CAD build for the part. Positions are in the model's coordinates, mm. A direction names the side the tool comes from. Give positions to 0.01 mm unless a question says otherwise; leave off trailing zeros. Answer as a JSON object with one key per item and string values.
from build123d import *

# Parameters (mm, degrees)
F2_R     = 7.9375
F3_DEPTH = 9.42848


with BuildPart() as f1:
    # F0 (on Front) → F1 (revolve)
    with BuildSketch(Plane.XZ):
        Polygon((-6.44752, 15.0876), (-6.44752, 11.176), (9.42748, 11.176), (9.42748, 16.34203), (7.903651, 16.319176), (7.48175, 44.45), (-3.61805, 44.45), (-3.61805, 15.0876), align=None)
    revolve(axis=Axis((0.264553, 0, 0), (1, 0, 0)))

    # F2 (on Right) → F3 (cut, through all)
    with BuildSketch(Plane.YZ):
        with Locations((0, 30.1625)):
            Circle(F2_R)
        with Locations((-30.1625, 0)):
            Circle(F2_R)
        with Locations((0, -30.1625)):
            Circle(F2_R)
        with Locations((30.1625, 0)):
            Circle(F2_R)
    extrude(amount=F3_DEPTH, mode=Mode.SUBTRACT)


solid = f1.part
Item 1: Probe line 1 (Y direction, x = 4.25, z = 0) (3 decimals); line 2 (Z direction, x = 4, y = 6). List the from-to ranges inside material, lowest first. Write a range as from..to.
Entries:
{"line 1": "-44.45..-38.1, -22.225..-11.176, 11.176..22.225, 38.1..44.45", "line 2": "-44.04..-35.36, -24.97..-9.43, 9.43..24.97, 35.36..44.04"}
Item 2: Which spindle directions (+Z, -Z, +X, -X, +Y, -Y) get a long thin tool onto all of the face, cutting with end or side? Do faces 5 (the cylindrical face through (1.854, -13.352, 42.397)), 6 (the flat face through (0, 0, -30)), 7 (the flat face through (-3.618, 19, -1)). Say none if no direction does.
Entries:
{"face 5": "+X, -X", "face 6": "+X", "face 7": "-X"}
Item 3: Flat gauge pins, fed straight in: P1, Ø3, axis at x = 1.5, z = -5.5, coming from the +Y side; P2, Ø1, axis at x = 2, z = 17, coming from the +Y side; P3, Ø8, axis at y = -8.5, z = -26.5, coming from the +X side. Where does each tip first touch, or does it go through?
Entries:
{"P1": "y = 44.27", "P2": "y = 41.27", "P3": "x = 7.79"}
Item 4: Mould opens along Y. For faces 1 (the conical face through (8.486, -4.904, 15.574)), 2 (the flat face through (9.427, 11, -3)), 3 (the flat face through (0, 30, 0)), 4 (the cylindrical face through (3.85, -1.72, -37.91)) say: +Y half, -Y half, draft (parallel to the pull), parting line (faces both ways), or undercut.
Entries:
{"face 1": "parting line", "face 2": "draft", "face 3": "undercut", "face 4": "undercut"}
Item 5: Cut at A-A (x = 1.75). State how many separate pieces and enclosed holes the cut face has, and give its area (3 significant figures).
Entries:
{"separate pieces": "1", "enclosed holes": "5", "area": "5,020 mm2"}
